```python
from build123d import *

# Parameters (mm, degrees)
SKETCH1_R           = 3
BOSS_EXTRUDE1_DEPTH = 80
SKETCH2_R           = 5.8
BOSS_EXTRUDE2_DEPTH = 4.3
FILLET1_R           = 1


with BuildPart() as part:
    # Sketch1 → Boss-Extrude1 (new body)
    with BuildSketch(Plane(origin=(0, 0, 0), x_dir=(1, 0, 0), z_dir=(0, 1, 0))):
        with Locations(Location((0, 0, 0), (0, 0, 270))):  # turned: the seam where the file's is
            Circle(SKETCH1_R)
    extrude(amount=BOSS_EXTRUDE1_DEPTH)

    # Sketch2 → Boss-Extrude2 (add)
    with BuildSketch(Plane(origin=(0, 80, 0), x_dir=(1, 0, 0), z_dir=(0, 1, 0))):
        with Locations(Location((0, 0, 0), (0, 0, 270))):  # turned: the seam where the file's is
            Circle(SKETCH2_R)
    extrude(amount=BOSS_EXTRUDE2_DEPTH)

    # Fillet1
    fillet1_edges = [part.edges().sort_by_distance(p)[0] for p in [
        (0, 80, -5.8),
        (0, 84.3, -5.8),
    ]]
    fillet(fillet1_edges, radius=FILLET1_R)


solid = part.part
```
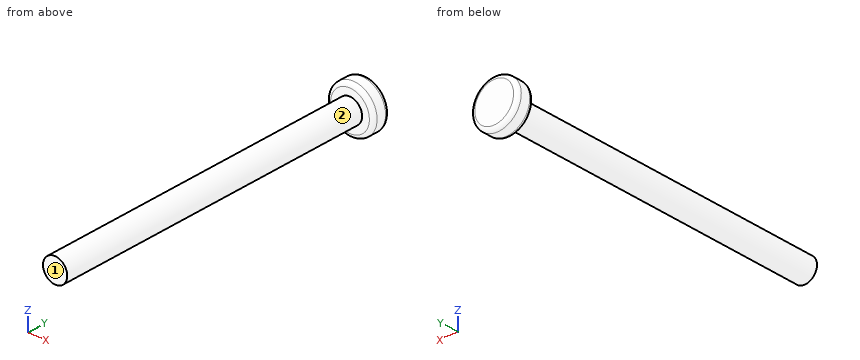
Build history of the part. All positions in model axes, mm. Face numbers are marked on the shaded views. A direction names the side the tool comes from. Round coordinates to 2 decimals unless told otherwise and drop trailing zeros. Order: outer loops, then holes, each group sorted by start corner. A loop starts at its lowest first (then second) coordinate and runs counter-clockwise, first axis right, second up. Notation, with made-up numbers: (-7, 39.25) - (40, 39.25) arc R29 ccw to (40, 77.25) - close; hole circle Ø4 at (55.5, 42.25). An arc over 180 degrees is marked (long way). Use a Markdown table: item, result.
1) Saw through at C-C on y = 78.5. Write the cut outline in (x, z).
Recorded:
| item | result |
|---|---|
| outline | circle Ø6 at (0, 0) |
2) Wall check: L1, parallel to Y at x = 4.25, z = -2; L2, parallel to X at y = 60, z = 0; L3, parallel to Z at x = 0.25, y = 66. Give the ranges that are in metal, low to high.
Recorded:
| item | result |
|---|---|
| L1 | y = 80 to 84.3 |
| L2 | x = -3 to 3 |
| L3 | z = -2.99 to 2.99 |
3) Tool access for the marked faces 1 and 2: list every direction of +Z, -Z, +X, -X, +Y, -Y with a clear straight run to the whole face (end or side of a thin tool).
Recorded:
| item | result |
|---|---|
| face 1 | +Z, -Z, +X, -X, -Y |
| face 2 | -Y |
4) Flat gauge pins, fed straight in: pin 1 Ø5 at (y, z) = (71.5, 3) entering from -X; pin 2 Ø6 at (x, y) = (2, 24) entering from -Z; pin 3 Ø1.5 at (y, z) = (70, 3) entering from -X. Where does each tip first touch, or does it go through?
Recorded:
| item | result |
|---|---|
| pin 1 | stops at x = -2.96 |
| pin 2 | stops at z = -3 |
| pin 3 | stops at x = -1.98 |
5) Saw through at A-A on z = 0. Write the cut outline in (x, y), and give its area (3 significant figures).
Recorded:
| item | result |
|---|---|
| outline | (-5.8, 81) arc R1 ccw to (-4.8, 80) - (-3, 80) - (-3, 0) - (3, 0) - (3, 80) - (4.8, 80) arc R1 ccw to (5.8, 81) - (5.8, 83.3) arc R1 ccw to (4.8, 84.3) - (-4.8, 84.3) arc R1 ccw to (-5.8, 83.3) - close |
| area | 529 mm² |
6) Saw through at B-B on x = 0. Write the cut outline in (y, z), and give its area (3 significant figures).
Recorded:
| item | result |
|---|---|
| outline | (0, -3) - (80, -3) - (80, -4.8) arc R1 ccw to (81, -5.8) - (83.3, -5.8) arc R1 ccw to (84.3, -4.8) - (84.3, 4.8) arc R1 ccw to (83.3, 5.8) - (81, 5.8) arc R1 ccw to (80, 4.8) - (80, 3) - (0, 3) - close |
| area | 529 mm² |
